```python
from build123d import *

# Parameters (mm, degrees)
F2_R     = 7.734325
F2_R_2   = 9.044999
F2_R_3   = 7.028051
F2_R_4   = 8.736696
F3_DEPTH = 76.2


with BuildPart() as f1:
    # F0 (on Front) → F1 (revolve)
    with BuildSketch(Plane.XZ):
        Polygon((0, 34.639813), (-21.368708, 34.639813), (-21.368708, 0), (9.222291, 0), (9.222291, 18.444577), (0, 18.444577), align=None)
    revolve(axis=Axis((-6.073209, 0, 0), (1, 0, 0)))

    # F2 (on Right) → F3 (join)
    with BuildSketch(Plane.YZ):
        with Locations((0, -34.850091)):
            Circle(F2_R)
        with Locations((-34.8488, 4.356261)):
            Circle(F2_R_2)
        with Locations((0, 29.912995)):
            Circle(F2_R_3)
        with Locations((31.21987, 0)):
            Circle(F2_R_4)
    extrude(amount=F3_DEPTH)


solid = f1.part
```
Check sheet for the modelled part. Datum: model origin and axes. Units: mm. A direction names the side the tool comes from. Round coordinates to 2 decimals unless told otherwise and drop trailing zeros. Write each loop counter-clockwise with the first axis right and the second up, starting at its lowest first coordinate (ties: lowest second). Pieces come first, ordered by that corner, then holes. Notation, with made-up numbers: M 20,81.25 L 50,81.25 A23 ccw 50,105.25 Z; hole C 5.25,35.5 d3. An arc over 180 degrees is marked long. Write item = value, one per line. Start each with the question number.
1. Section check C-C, the plane z = 0. Record the cut outline in (x, y).
2. Section check D-D, the plane y = 29. Record the cut outline in (x, z).
3. Section check B-B, the plane x = 4. Record the cut outline in (y, z) (3 decimals), then the cut area to 3 significant figures.
4. Section check A-A, the plane y = 0. Record the cut outline in (x, z), then the cut area to 3 significant figures.
5. Release check for a two-part mould opening along Z. For faces 1 (the flat face through (9.222, 0, 0)), 2 (the flat face through (76.2, 0, -35)), 3 (the cylindrical face through (37.57, 22.49, 0.38)) record: pulls with the +Z half, pulls with the -Z half, needs draft (parallel to the pull), parting line crosses it, or undercut.
6. Tool access check on faces 4 (the cylindrical face through (-10.83, -29.21, 18.62)), 5 (the flat face through (76.2, -35, 4)), 6 (the cylindrical face through (37.57, 3.78, 35.84)). Record the directions out of +Z, -Z, +X, -X, +Y, -Y that give a thin tool (end or side, any length) a straight path to the whole face; none if there is none.
7. Gauge pin test, flat ends, axial feed: pin 1 (18.5 mm diameter, centred on y = 4.5, z = 6.5, fed in from +X); pin 2 (1 mm diameter, centred on y = -19, z = -21, fed in from +X); pin 3 (1 mm diameter, centred on x = 61.5, y = -7.5, fed in from -Z). Record the tip position at first contact, or that the pin passes through.
8. Scan lines: line 1 (Y direction, x = 6.5, z = 0.5); line 2 (X direction, y = -24, z = 24); line 3 (Z direction, x = 53, y = -1.5). Record each from-to range of solid material in increasing order. Write a range as [from, to].
Results found:
q1.outline = M -21.37,-34.64 L 0,-34.64 L 0,-42.78 L 76.2,-42.78 L 76.2,-26.92 L 0,-26.92 L 0,-18.44 L 9.22,-18.44 L 9.22,18.44 L 0,18.44 L 0,22.48 L 76.2,22.48 L 76.2,39.96 L 0,39.96 L 0,34.64 L -21.37,34.64 Z
q2.outline = M -21.37,-18.95 L 0,-18.95 L 0,-8.45 L 76.2,-8.45 L 76.2,8.45 L 0,8.45 L 0,18.95 L -21.37,18.95 Z
q3.outline = C -34.849,4.356 d18.09; C 0,0 d36.889; C 0,-34.85 d15.469; C 0,29.913 d14.056; C 31.22,0 d17.473
q3.area = 1,910 mm^2
q4.outline = M -21.37,-34.64 L 0,-34.64 L 0,-42.58 L 76.2,-42.58 L 76.2,-27.12 L 0,-27.12 L 0,-18.44 L 9.22,-18.44 L 9.22,18.44 L 0,18.44 L 0,22.88 L 76.2,22.88 L 76.2,36.94 L 0,36.94 L 0,34.64 L -21.37,34.64 Z
q4.area = 4,070 mm^2
q5.face_1 = undercut
q5.face_2 = needs draft
q5.face_3 = parting line crosses it
q6.face_4 = -X
q6.face_5 = +Z, -Z, +X, +Y, -Y
q6.face_6 = +X
q7.pin_1 = 9.22
q7.pin_2 = 0
q7.pin_3 = -38.14
q8.line_1 = [-43.03, -26.67], [-18.44, 18.44], [22.5, 39.94]
q8.line_2 = [-21.37, 0]
q8.line_3 = [-42.44, -27.26], [23.05, 36.78]
